```python
from build123d import *

# Parameters (mm, degrees)
F3_D     = 6.35
F4_R     = 0.79375
F5_DEPTH = 3.96875


with BuildPart() as f1:
    # F0 (on Right) → F1 (revolve)
    with BuildSketch(Plane.YZ):
        Polygon((-2.38125, 9.525), (-2.38125, 0), (0, 0), (2.38125, 0), (2.38125, 9.525), (1.5875, 9.525), (1.5875, 7.9375), (-1.5875, 7.9375), (-1.5875, 9.525), align=None)
    revolve(axis=Axis((0, 1.190625, 0), (0, -1, 0)))

    # F3 (through all)
    with Locations(Plane.XZ.offset(2.38125)):
        with Locations((0, 3.175)):
            Hole(F3_D / 2)

    # F4 (on face) → F5 (join)
    with BuildSketch(Plane.XZ.offset(2.38125)):
        with Locations((0, -4.7625)):
            Circle(F4_R)
    extrude(amount=F5_DEPTH)


solid = f1.part
```
Model file for the job. Use its own axes, mm. A direction names the side the tool comes from. Coordinates: 2 decimals unless noted, no trailing zeros. Order: outer loops, then holes, each group sorted by start corner. A loop starts at its lowest first (then second) coordinate and runs counter-clockwise, first axis right, second up. Notation, with made-up numbers: M -19,68 L 6,68 A15 cw 6,75 Z; hole C 13.5,40.25 d5. An arc over 180 degrees is marked long. Answer as CSV lines item,"result".
(1) Band-saw the part on B-B, the plane z = 0.75. List the corners of the cut face in (x, y).
Geometry says:
outline,"M -9.5,-2.38 L -2.05,-2.38 L -2.05,2.38 L -9.5,2.38 L -9.5,1.59 L -7.9,1.59 L -7.9,-1.59 L -9.5,-1.59 Z; M 2.05,-2.38 L 9.5,-2.38 L 9.5,-1.59 L 7.9,-1.59 L 7.9,1.59 L 9.5,1.59 L 9.5,2.38 L 2.05,2.38 Z"
(2) 3-axis set-ups, long thin cutter, end or side, ignore diameter. For faces 1 (the flat face through (-8, -1.588, 2)), 2 (the cylindrical face through (0.757, -4.338, -4.524)), 3 (the cylindrical face through (5.796, 1.979, -7.559)): which of +Z, -Z, +X, -X, +Y, -Y reach the whole face in a straight line?
Geometry says:
face 1,"none"
face 2,"-Y"
face 3,"+Y, -Y"
(3) Flat gauge pins, fed straight in: pin 1 (5 mm diameter, centred on y = -1.5, z = 6, fed in from +X); pin 2 (6 mm diameter, centred on x = -4.5, z = 7.5, fed in from -Y); pin 3 (4 mm diameter, centred on x = 3, y = -2, fed in from +Z). Where does each tip first touch, or does it go through?
Geometry says:
pin 1,"stops at x = 8.86"
pin 2,"stops at y = -2.38"
pin 3,"stops at z = 9.47"
(4) Wall check: line 1 along Z through (x, y) = (0, 1.45); line 2 along Y through (x, z) = (-8.5, -3.75); line 3 along Z through (x, y) = (-1.5, 1.5). Give the ranges that are in metal, low to high.
Geometry says:
line 1,"z = -7.94 to 0, 6.35 to 7.94"
line 2,"y = -2.38 to -1.59, 1.59 to 2.38"
line 3,"z = -7.79 to 0.38, 5.97 to 7.79"
(5) Band-saw the part on D-D, the plane x = -4.5. List the corners of the cut face in (y, z), then the cut area to 3 significant figures.
Geometry says:
outline,"M -2.38,-8.39 L -1.59,-8.39 L -1.59,-6.54 L 1.59,-6.54 L 1.59,-8.39 L 2.38,-8.39 L 2.38,8.39 L 1.59,8.39 L 1.59,6.54 L -1.59,6.54 L -1.59,8.39 L -2.38,8.39 Z"
area,"68.2 mm2"
(6) Band-saw the part on C-C, the plane z = -1.5. List the corners of the cut face in (x, y).
Geometry says:
outline,"M -9.41,-2.38 L 9.41,-2.38 L 9.41,-1.59 L 7.79,-1.59 L 7.79,1.59 L 9.41,1.59 L 9.41,2.38 L -9.41,2.38 L -9.41,1.59 L -7.79,1.59 L -7.79,-1.59 L -9.41,-1.59 Z"
(7) Pull direction Z, two halves, no side cores. Call faces 4 (the cylindrical face through (0.413, 0.033, 6.323)), 5 (the flat face through (2, -2.381, 0)), 6 (the cylindrical face through (5.796, -1.99, -7.559)): +Z half, -Z half, draft (parallel to the pull), parting line (faces both ways), or undercut.
Geometry says:
face 4,"undercut"
face 5,"draft"
face 6,"parting line"
